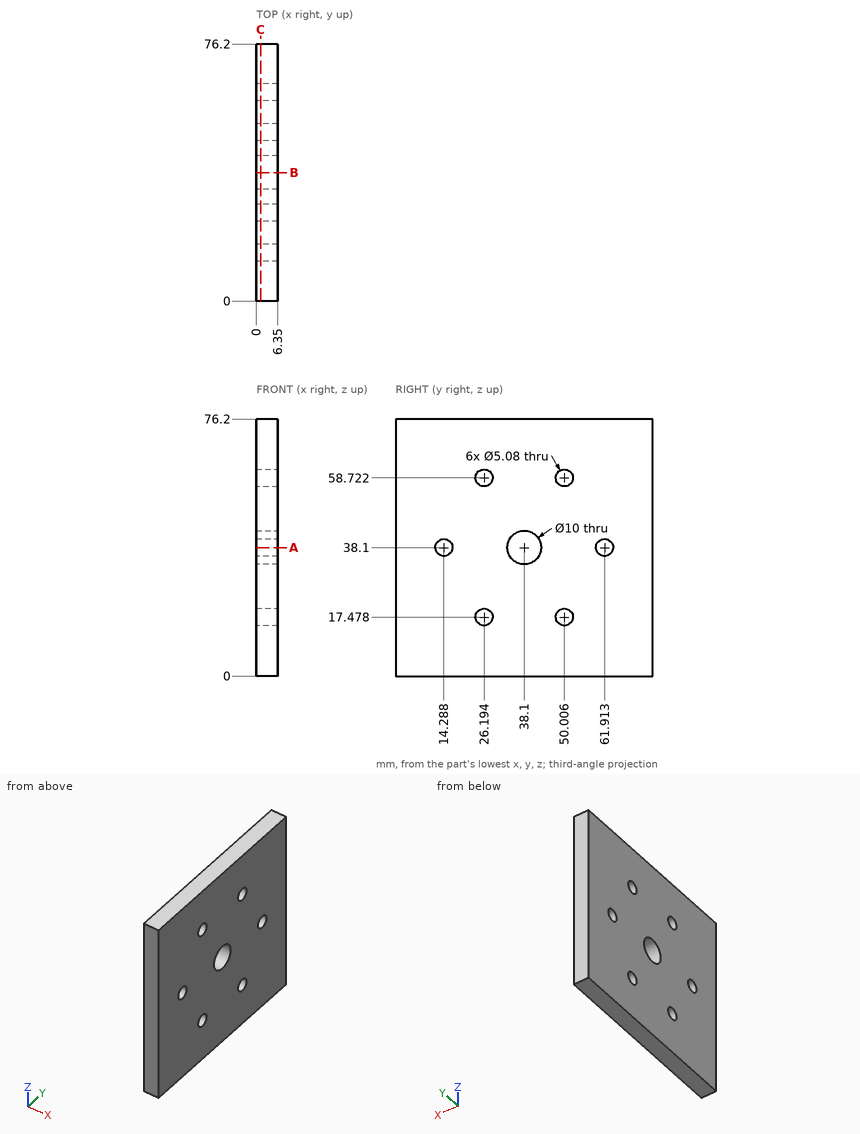
Geometry check sheet. Reference: drawing and pictorial views, mm from the part's lowest x, y, z. Round coordinates to 2 decimals unless told otherwise and drop trailing zeros. Order: outer loops, then holes, each group sorted by start corner. A loop starts at its lowest first (then second) coordinate and runs counter-clockwise, first axis right, second up. Notation, with made-up numbers: M 67,28 L 72,28 A37 cw 72,66 Z; hole C 8,86 d8. An arc over 180 degrees is marked long. Answer as CSV lines item,"result".
1) Thickness scan on probe 1 along Z at (x, y) = (0.5, 26.5); probe 2 along Y at (x, z) = (4.5, 38.1); probe 3 along Z at (x, y) = (2.5, 50). Record the ranges inside material, lowest first. Write a range as [from, to].
Entries:
probe 1,"[0, 14.96], [20, 56.2], [61.24, 76.2]"
probe 2,"[0, 11.75], [16.83, 33.1], [43.1, 59.37], [64.45, 76.2]"
probe 3,"[0, 14.94], [20.02, 56.18], [61.26, 76.2]"
2) Gauge pin test, flat end, axial feed: pin 1 Ø11.5 at (y, z) = (38.1, 38.1) entering from -X. Record the tip position at first contact, or that the pin passes through.
Entries:
pin 1,"x = 0"
3) Sectioned sample at C-C on x = 1.25. Record the cut outline in (y, z), and give its area (3 significant figures).
Entries:
outline,"M 0,0 L 76.2,0 L 76.2,76.2 L 0,76.2 Z; hole C 14.29,38.1 d5.08; hole C 26.19,17.48 d5.08; hole C 26.19,58.72 d5.08; hole C 38.1,38.1 d10; hole C 50.01,17.48 d5.08; hole C 50.01,58.72 d5.08; hole C 61.91,38.1 d5.08"
area,"5,610 mm2"
4) Sectioned sample at A-A on z = 38.1. Record the cut outline in (x, y).
Entries:
outline,"M 0,0 L 6.35,0 L 6.35,11.75 L 0,11.75 Z; M 0,16.83 L 6.35,16.83 L 6.35,33.1 L 0,33.1 Z; M 0,43.1 L 6.35,43.1 L 6.35,59.37 L 0,59.37 Z; M 0,64.45 L 6.35,64.45 L 6.35,76.2 L 0,76.2 Z"
5) Sectioned sample at B-B on y = 38.1. Record the cut outline in (x, z).
Entries:
outline,"M 0,0 L 6.35,0 L 6.35,33.1 L 0,33.1 Z; M 0,43.1 L 6.35,43.1 L 6.35,76.2 L 0,76.2 Z"
